Autodesk Inventor part; units mm, degrees
ref_plane "YZ Plane" through (0, 0, 0) normal (1, 0, 0) x (0, 1, 0)
ref_plane "XZ Plane" through (0, 0, 0) normal (0, 1, 0) x (-1, 0, 0)
ref_plane "XY Plane" through (0, 0, 0) normal (0, 0, 1) x (1, 0, 0)
sketch "Sketch1" plane through (0, 0, 0) normal (0, 0, 1) x (1, 0, 0)
  circle A0 centre (0, 0) radius 7.975
  circle A1 centre (0, 0) radius 6.05
  dimension "d0" = 15.95
  dimension "d1" = 12.1
extrude "Extrusion1" add sketch "Sketch1" along normal blind 10
sketch "Sketch2" plane through (0, 0, 10) normal (0, 0, 1) x (1, 0, 0)
  circle A0 centre (0, 0) radius 7.975
  line L0 (-6.225, 6.225) -> (6.225, 6.225)
  line L1 (6.225, 6.225) -> (6.225, -6.225)
  line L2 (6.225, -6.225) -> (-6.225, -6.225)
  line L3 (-6.225, -6.225) -> (-6.225, 6.225)
  line L4 (-6.225, 6.225) -> (6.225, -6.225) construction
  line L5 (6.225, 6.225) -> (-6.225, -6.225) construction
  line L6 (-8.5, 0.875) -> (8.5, 0.875)
  line L7 (8.5, 0.875) -> (8.5, -0.875)
  line L8 (8.5, -0.875) -> (-8.5, -0.875)
  line L9 (-8.5, -0.875) -> (-8.5, 0.875)
  line L10 (-8.5, 0.875) -> (8.5, -0.875) construction
  line L11 (8.5, 0.875) -> (-8.5, -0.875) construction
  circle A1 centre (0, 0) radius 12
  point P0 (4.985, -6.225)
  point P1 (-4.985, -6.225)
  point P2 (7.9269, -0.875)
  point P3 (6.225, -0.875)
  point P4 (6.225, -4.985)
  point P5 (-6.225, -0.875)
  point P6 (-7.9269, -0.875)
  point P7 (-6.225, -4.985)
  point P8 (6.225, 0.875)
  point P9 (7.9269, 0.875)
  point P10 (6.225, 4.985)
  point P11 (-7.9269, 0.875)
  point P12 (-6.225, 0.875)
  point P13 (-6.225, 4.985)
  point P14 (-4.985, 6.225)
  point P15 (4.985, 6.225)
  dimension "d4" = 12.45
  dimension "d5" = 12.45
  dimension "d6" = 17
  dimension "d7" = 1.75
  dimension "d10" = 24
extrude "Extrusion2" add sketch "Sketch2" along normal blind 7 contours L6 L1 A0 | A0 L1 L8 | L0 A0 | L6 A0 L3 | A0 L2 | L3 A0 L8 | A1
sketch "Sketch3" plane through (0, 0, 10) normal (0, 0, -1) x (-1, 0, 0)
  circle A0 centre (0, 0) radius 7.975
  circle A1 centre (0, 0) radius 12
extrude "Extrusion3" add sketch "Sketch3" along normal blind 0.2
chamfer "Chamfer1" distance 2 angle 45 1 edges at (-7.975, 0, 9.8)
chamfer "Chamfer2" distance 2 angle 45 1 edges at (12, 0, 9.8)
properties part number "CouplerAdapter"
The model under review builds one solid part; all positions refer to its coordinate system, in mm. A direction names the side the tool comes from. Coordinates: 2 decimals unless noted, no trailing zeros. Order: outer loops, then holes, each group sorted by start corner. A loop starts at its lowest first (then second) coordinate and runs counter-clockwise, first axis right, second up. Notation, with made-up numbers: (42.25, 19.5) -> (81.25, 19.5) arc R23 ccw to (81.25, 45.5) -> close; hole circle Ø9 at (71.25, -22.5). An arc over 180 degrees is marked (long way). Answer in a Markdown table with one row per item.
(1) Consider section B-B (z = 8.75). Write out the cut boundary in (x, y) (3 decimals).
Answers:
| item | result |
|---|---|
| outline | circle Ø17.85 at (0, 0); hole circle Ø12.1 at (0, 0) |
(2) Wall thickness on line 1 along Y through (x, z) = (0, 5) (3 decimals); line 2 along Z through (x, y) = (-6, 1.5); line 3 along X through (y, z) = (-6, 11.5) (3 decimals): over which ranges is each line inside the solid? List them lowest first.
Answers:
| item | result |
|---|---|
| line 1 | -7.975 to -6.05, 6.05 to 7.975 |
| line 2 | 0 to 10 |
| line 3 | -10.044 to -6.225, 6.225 to 10.044 |
(3) Insertion check: pin 1 (1 mm diameter, centred on x = -4.5, z = 10, fed in from +Y); pin 2 (1.9 mm diameter, centred on y = -0.5, z = 13, fed in from -X); pin 3 (10 mm diameter, centred on y = -0.5, z = 3, fed in from +X); pin 4 (0.7 mm diameter, centred on x = -8, z = 15, fed in from -Y). Each pin has a flat end and moves straight along its axis. Give the tip position at first contact, or say it passes through.
Answers:
| item | result |
|---|---|
| pin 1 | y = 9.75 |
| pin 2 | x = -12 |
| pin 3 | x = 8.17 |
| pin 4 | y = -9.25 |
(4) Consider section A-A (z = 3.25). Write out the cut boundary in (x, y) (3 decimals), plus the area to 3 significant figures.
Answers:
| item | result |
|---|---|
| outline | circle Ø15.95 at (0, 0); hole circle Ø12.1 at (0, 0) |
| area | 84.8 mm² |
(5) Machinability: for faces 1 (the cylindrical face through (7.607, -2.395, 3.845)), 2 (the flat face through (-7, -0.875, 13)), 3 (the cylindrical face through (5.589, 2.317, 4.93)), which of the approach directions +Z, -Z, +X, -X, +Y, -Y give a long, thin tool a straight path to every point of the face, cutting with its end or side? Answer none if there is none.
Answers:
| item | result |
|---|---|
| face 1 | -Z |
| face 2 | +Z |
| face 3 | +Z, -Z |
